Can you work these out from the model? Positions are in its coordinate system, mm. Round coordinates to 2 decimals unless told otherwise and drop trailing zeros. Loops run counter-clockwise (first coordinate to the right, second up) from the corner with the lowest first, then second, coordinate; pieces in that order, holes last.
(1) If I drill on line 1 along Y through (x, z) = (-46, -1.1); line 2 along Y through (x, z) = (-18, -1.2); line 3 along X through (y, z) = (48, 1.5), over which ranges is the centre line in solid material (lowest first)?
(2) I want a section at C-C on z = -0.15. Write out the boundary of the cut face in (x, y) (3 decimals).
(3) I want a section at B-B on y = 0. Write out the boundary of the cut face in (x, z).
(4) I want a section at A-A on x = 31. Write out the boundary of the cut face in (y, z) (3 decimals).
(5) I want a section at D-D on x = -12.5. Write out the boundary of the cut face in (y, z), plus the area to 3 significant figures.
(6) Will these pins go through, and if not, where does the flat tip stop? pin 1 Ø2 at (y, z) = (-1.5, -0.5) entering from +X; pin 2 Ø0.8 at (x, z) = (32, -0.5) entering from +Y; pin 3 Ø0.8 at (x, z) = (-54, -0.5) entering from +Y.
from build123d import *
from OCP.BRepFilletAPI import BRepFilletAPI_MakeChamfer

# Parameters (mm, degrees)
SKETCH1_R           = 5
SKETCH1_R_2         = 2.83
SKETCH1_R_3         = 3.25
SKETCH1_W           = 9.2
SKETCH1_H           = 3.53
SKETCH1_H_2         = 3.4
BOSS_EXTRUDE1_DEPTH = 2
BOSS_EXTRUDE2_DEPTH = 2
CHAMFER1_SIZE       = 0.5
CHAMFER1_SIZE2      = 1.5
CHAMFER2_SIZE       = 1.5
CHAMFER2_SIZE2      = 0.5


with BuildPart() as part:
    # Sketch1 → Boss-Extrude1 (new, symmetric)
    with BuildSketch(Plane.XY):
        Polygon((-86, -30), (-86, 30), (52.3, 30), (52.3, 13), (47.3, 13), (47.3, -13), (52.3, -13), (52.3, -30), align=None)
        with Locations((-46, 0)):
            Circle(SKETCH1_R, mode=Mode.SUBTRACT)
        with Locations((25, -24)):
            Circle(SKETCH1_R_2, mode=Mode.SUBTRACT)
        with Locations((-12.5, 24.5)):
            Circle(SKETCH1_R_3, mode=Mode.SUBTRACT)
        with Locations((30.35, -5)):
            Rectangle(SKETCH1_W, SKETCH1_H, mode=Mode.SUBTRACT)
        with Locations((-52.65, -12)):
            Rectangle(SKETCH1_W, SKETCH1_H_2, mode=Mode.SUBTRACT)
    extrude(amount=BOSS_EXTRUDE1_DEPTH, both=True)

    # Sketch2 → Boss-Extrude2 (add, symmetric)
    with BuildSketch(Plane.XY):
        Polygon((-86, 30), (52.3, 30), (52.3, 55), (37.3, 55), (23.157864376, 40.857864376), (-56.857864376, 40.857864376), (-71, 55), (-86, 55), align=None)
    extrude(amount=BOSS_EXTRUDE2_DEPTH, both=True)

    # Chamfer1
    chamfer1_edges = [part.edges().sort_by_distance(p)[0] for p in [
        (-57.25, -12, 2),
        (-52.65, -13.7, 2),
        (-48.05, -12, 2),
        (-52.65, -10.3, 2),
        (-15.75, 24.5, 2),
        (-51, 0, 2),
        (25.75, -5, 2),
        (30.35, -6.765, 2),
        (34.95, -5, 2),
        (30.35, -3.235, 2),
        (22.17, -24, 2),
    ]]
    chamfer1_side = [part.faces().sort_by_distance(p)[0] for p in [
        (-17.641163969, 8.221234178, 2),
    ]]
    chamfer(chamfer1_edges, length=CHAMFER1_SIZE, length2=CHAMFER1_SIZE2, reference=chamfer1_side[0])

    # Chamfer2: one chamfer whose edges measure the first distance from different faces: ONE call of the kernel's chamfer builder (chamfer() names one face for all edges)
    chamfer2_edges_1 = [part.edges().sort_by_distance(p)[0] for p in [
        (49.8, -13, 2),
    ]]
    chamfer2_side_1 = [part.faces().sort_by_distance(p)[0] for p in [
        (49.8, -13, 0),
    ]]
    chamfer2_edges_2 = [part.edges().sort_by_distance(p)[0] for p in [
        (47.3, 0, 2),
    ]]
    chamfer2_side_2 = [part.faces().sort_by_distance(p)[0] for p in [
        (47.3, 0, 0),
    ]]
    chamfer2_edges_3 = [part.edges().sort_by_distance(p)[0] for p in [
        (49.8, 13, 2),
    ]]
    chamfer2_side_3 = [part.faces().sort_by_distance(p)[0] for p in [
        (49.8, 13, 0),
    ]]
    chamfer2 = BRepFilletAPI_MakeChamfer(part.part.solid().wrapped)
    for e in chamfer2_edges_1:
        chamfer2.Add(CHAMFER2_SIZE, CHAMFER2_SIZE2, e.wrapped, chamfer2_side_1[0].wrapped)  # the first distance lies on this face
    for e in chamfer2_edges_2:
        chamfer2.Add(CHAMFER2_SIZE, CHAMFER2_SIZE2, e.wrapped, chamfer2_side_2[0].wrapped)  # the first distance lies on this face
    for e in chamfer2_edges_3:
        chamfer2.Add(CHAMFER2_SIZE, CHAMFER2_SIZE2, e.wrapped, chamfer2_side_3[0].wrapped)  # the first distance lies on this face
    add(Compound.cast(chamfer2.Shape()), mode=Mode.REPLACE)


solid = part.part
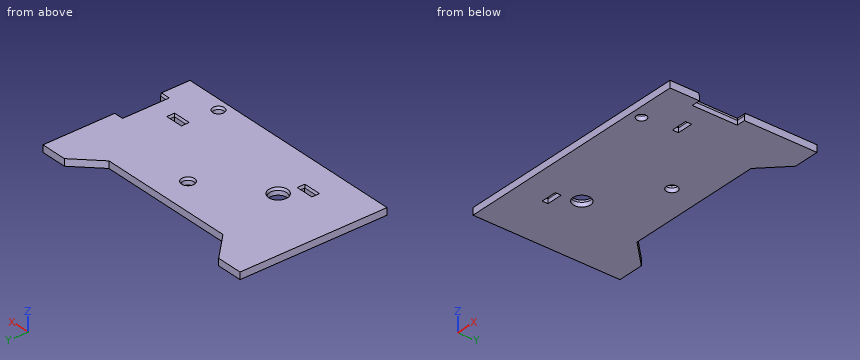
Filled sheet:
1. line 1: y = -30 to -5, 5 to 40.86
1. line 2: y = -30 to 40.86
1. line 3: x = -86 to -64, 30.3 to 52.3
2. outline: (-86, -30) - (52.3, -30) - (52.3, -13) - (47.3, -13) - (47.3, 13) - (52.3, 13) - (52.3, 55) - (37.3, 55) - (23.158, 40.858) - (-56.858, 40.858) - (-71, 55) - (-86, 55) - close; hole (-57.25, -13.7) - (-48.05, -13.7) - (-48.05, -10.3) - (-57.25, -10.3) - close; hole circle Ø10 at (-46, 0); hole circle Ø6.5 at (-12.5, 24.5); hole circle Ø5.66 at (25, -24); hole (25.75, -6.765) - (34.95, -6.765) - (34.95, -3.235) - (25.75, -3.235) - close
3. outline: (-86, -2) - (-51, -2) - (-51, 0.5) - (-51.5, 2) - (-86, 2) - close; (-41, -2) - (47.3, -2) - (47.3, 0.5) - (46.8, 2) - (-40.5, 2) - (-41, 0.5) - close
4. outline: (-30, -2) - (-6.765, -2) - (-6.765, 0.5) - (-7.265, 2) - (-30, 2) - close; (-3.235, -2) - (48.7, -2) - (48.7, 2) - (-2.735, 2) - (-3.235, 0.5) - close
5. outline: (-30, -2) - (21.25, -2) - (21.25, 0.5) - (20.75, 2) - (-30, 2) - close; (27.75, -2) - (40.86, -2) - (40.86, 2) - (28.25, 2) - (27.75, 0.5) - close
5. area: 257 mm2
6. pin 1: stops at x = 47.3
6. pin 2: stops at y = 50.1
6. pin 3: stops at y = 40.86
